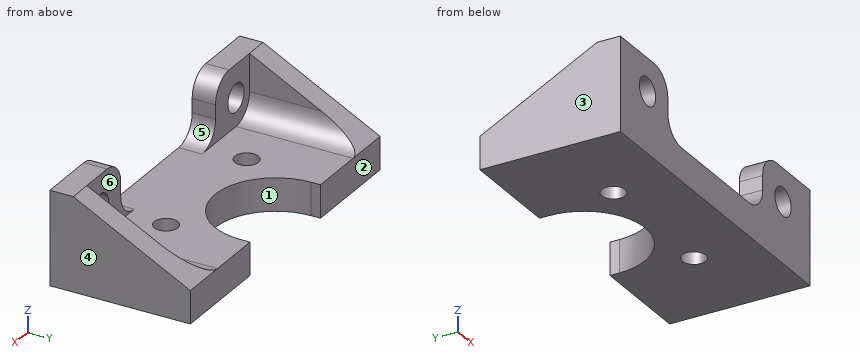
```python
from build123d import *

# Parameters (mm, degrees)
SKETCH1_R           = 2.5
BOSS_EXTRUDE1_DEPTH = 20
CUT_EXTRUDE1_DEPTH  = 71
SKETCH3_R           = 3
CUT_EXTRUDE2_DEPTH  = 31
CUT_EXTRUDE3_START  = -5
CUT_EXTRUDE3_DEPTH  = 26
FILLET1_R           = 5


with BuildPart() as part:
    # Sketch1 → Boss-Extrude1 (new body)
    with BuildSketch(Plane.XY):
        with BuildLine():
            Line((0, 0), (0, 5))
            Line((0, 5), (0, 30))
            Line((0, 30), (22, 30))
            Line((22, 30), (22, 28))
            ThreePointArc((22, 28), (35, 15), (48, 28))
            Line((48, 28), (48, 30))
            Line((48, 30), (70, 30))
            Line((70, 30), (70, 5))
            Line((70, 5), (70, 0))
            Line((70, 0), (0, 0))
        make_face()
        with Locations((20.150757595, 13.150757595)):
            Circle(SKETCH1_R, mode=Mode.SUBTRACT)
        with Locations((49.849242405, 13.150757595)):
            Circle(SKETCH1_R, mode=Mode.SUBTRACT)
    extrude(amount=BOSS_EXTRUDE1_DEPTH)

    # Sketch2 → Cut-Extrude1 (cut, through all)
    with BuildSketch(Plane(origin=(70, 0, 0), x_dir=(0, 0, -1), z_dir=(1, 0, 0))):
        Polygon((-7, 30), (-20, 5), (-20, 30), align=None)
    extrude(amount=-CUT_EXTRUDE1_DEPTH, mode=Mode.SUBTRACT)

    # Sketch3 → Cut-Extrude2 (cut, through all)
    with BuildSketch(Plane.XZ):
        with Locations(Location((10, 13, 0), (0, 0, 270))):  # turned: the seam where the file's is
            Circle(SKETCH3_R)
        with Locations(Location((60, 13, 0), (0, 0, 270))):  # turned: the seam where the file's is
            Circle(SKETCH3_R)
        with BuildLine():
            Line((17.5, 20), (52.5, 20))
            Line((52.5, 20), (52.5, 12))
            ThreePointArc((52.5, 12), (51.035533906, 8.464466094), (47.5, 7))
            Line((47.5, 7), (22.5, 7))
            ThreePointArc((22.5, 7), (18.964466094, 8.464466094), (17.5, 12))
            Line((17.5, 12), (17.5, 20))
        make_face()
    extrude(amount=-CUT_EXTRUDE2_DEPTH, mode=Mode.SUBTRACT)

    # Sketch4 → Cut-Extrude3 (cut, through all)
    with BuildSketch(Plane.XZ.offset(CUT_EXTRUDE3_START)):
        with BuildLine():
            Line((65, 12), (65, 20))
            Line((65, 20), (5, 20))
            Line((5, 20), (5, 12))
            ThreePointArc((5, 12), (6.464466094, 8.464466094), (10, 7))
            Line((10, 7), (60, 7))
            ThreePointArc((60, 7), (63.535533906, 8.464466094), (65, 12))
        make_face()
    extrude(amount=-CUT_EXTRUDE3_DEPTH, mode=Mode.SUBTRACT)

    # Fillet1
    fillet1_edges = [part.edges().sort_by_distance(p)[0] for p in [
        (17.5, 2.5, 20),
        (52.5, 2.5, 20),
    ]]
    fillet(fillet1_edges, radius=FILLET1_R)


solid = part.part
```
Model file for the job. Use its own axes, mm. Face numbers are marked on the shaded views. A direction names the side the tool comes from. Give positions to 0.01 mm unless a question says otherwise; leave off trailing zeros. Order: outer loops, then holes, each group sorted by start corner. A loop starts at its lowest first (then second) coordinate and runs counter-clockwise, first axis right, second up.
1) Wall check: probe 1 along X at (y, z) = (2.7, 13); probe 2 along Z at (x, y) = (43, 1.5); probe 3 along Y at (x, z) = (10.5, 8.25). Give the ranges that are in metal, low to high.
2) Mould opens along X. For the marked faces 1, 2 and 3 say: +X half, -X half, draft (parallel to the pull), parting line (faces both ways), or undercut.
3) 3-axis set-ups, long thin cutter, end or side, ignore diameter. For the marked faces 4, 5 and 6: which of +Z, -Z, +X, -X, +Y, -Y reach the whole face in a straight line?
4) Pin check, flat tips, straight feed: pin 1 (10.5 mm diameter, centred on x = 14.5, z = 10.5, fed in from +Y); pin 2 (7 mm diameter, centred on x = 60, z = 13, fed in from +Y); pin 3 (1 mm diameter, centred on x = 58, y = 24, fed in from +Z). Stop position of each tip, or through.
5) Saw through at A-A, the plane y = 2.25. Write the cut outline in (x, z).
6) Saw through at B-B, the plane z = 17. Write the cut outline in (x, y), then the cut area to 3 significant figures.
7) Saw through at D-D, the plane z = 13. Write the cut outline in (x, y).
8) Saw through at C-C, the plane x = 49.5. Write the cut outline in (y, z), then the cut area to 3 significant figures.
Computed:
1. probe 1: x = 0 to 7, 13 to 17.5, 52.5 to 57, 63 to 70
1. probe 2: z = 0 to 7
1. probe 3: y = 0 to 5
2. face 1: undercut
2. face 2: draft
2. face 3: -X half
3. face 4: +Z, -Z, +X, +Y, -Y
3. face 5: +Z, +Y, -Y
3. face 6: +Z, +Y
4. pin 1: stops at y = 30
4. pin 2: stops at y = 5
4. pin 3: stops at z = 7
5. outline: (0, 0) - (70, 0) - (70, 20) - (57.5, 20) arc R5 ccw to (52.5, 15) - (52.5, 12) arc R5 cw to (47.5, 7) - (22.5, 7) arc R5 cw to (17.5, 12) - (17.5, 15) arc R5 ccw to (12.5, 20) - (0, 20) - close; hole circle Ø6 at (10, 13); hole circle Ø6 at (60, 13)
6. outline: (0, 0) - (17.08, 0) - (17.08, 5) - (5, 5) - (5, 10.77) - (0, 10.77) - close; (52.92, 0) - (70, 0) - (70, 10.77) - (65, 10.77) - (65, 5) - (52.92, 5) - close
6. area: 229 mm2
7. outline: (0, 0) - (7, 0) - (7, 5) - (5, 5) - (5, 18.46) - (0, 18.46) - close; (13, 0) - (17.5, 0) - (17.5, 5) - (13, 5) - close; (52.5, 0) - (57, 0) - (57, 5) - (52.5, 5) - close; (63, 0) - (70, 0) - (70, 18.46) - (65, 18.46) - (65, 5) - (63, 5) - close
8. outline: (0, 0) - (10.68, 0) - (10.68, 7) - (5, 7) - (5, 7.42) - (0, 7.42) - close; (15.63, 0) - (30, 0) - (30, 7) - (15.63, 7) - close
8. area: 177 mm2
